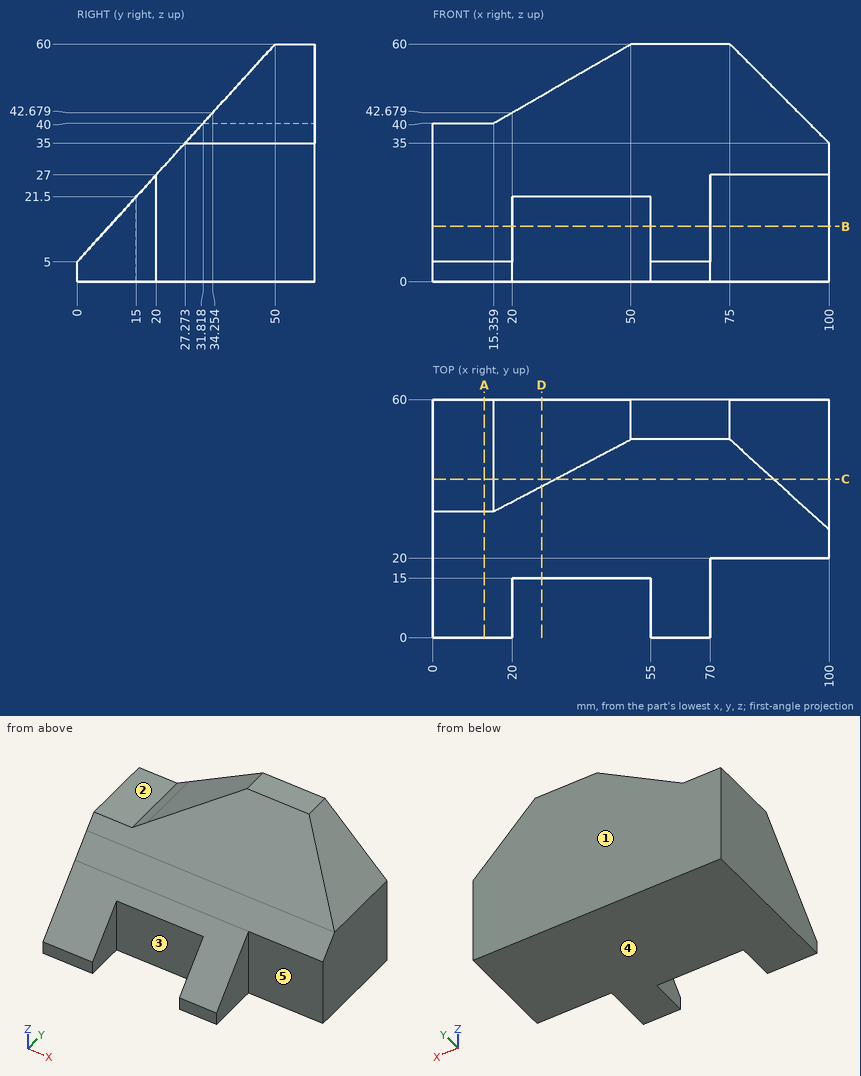
Answer from the drawing. Dimensions are ordinates in mm from the lowest x, y and z of the part. A direction names the side the tool comes from. Round coordinates to 2 decimals unless told otherwise and drop trailing zeros. Write each loop counter-clockwise with the first axis right and the second up, starting at its lowest first coordinate (ties: lowest second). Pieces come first, ordered by that corner, then holes. Notation, with made-up numbers: (-7.5, -16) -> (29.5, -16) arc R29 cw to (29.5, 11) -> close; hole circle Ø1 at (88.5, 51.5). An arc over 180 degrees is marked (long way). Answer in a Markdown table with one row per item. Add a question column.
1) Find section D-D, the plane x = 27.5. Determine the outline of the cut face in (y, z), and give its area (3 significant figures).
2) Given P1, Ø5, axis at x = 10.5, y = 19.5, coming from the -Z side; P2, Ø8, axis at x = 83.5, z = 15.5, coming from the -Y side; P3, Ø2, axis at x = 24.5, y = 18, coming from the +Z side; P4, Ø4.5, axis at x = 9.5, y = 43, coming from the +Z side, each flat-ended and moving along its own axis, determine where each tip first touches the part or whether it passes through.
3) Find section B-B, the plane z = 14. Determine the outline of the cut face in (x, y).
4) Find section C-C, the plane y = 40. Determine the outline of the cut face in (x, z), and give its area (3 significant figures).
5) Consider line 1 (Y direction, x = 25, z = 18.5); line 2 (Y direction, x = 33, z = 49); line 3 (Z direction, x = 52, y = 20). Determine where each line is inside the solid, lowest interval first.
6) Find section A-A, the plane x = 13. Determine the outline of the cut face in (y, z), and give its area (3 significant figures).
7) Which of the six approach directions +Z, -Z, +X, -X, +Y, -Y give full straight-line access (tool end or side, diameter ignored) to the marked faces 1, 2, 3, 4 and 5?
Findings below:
| question | item | result |
|---|---|---|
| 1 | outline | (15, 0) -> (60, 0) -> (60, 47.01) -> (38.19, 47.01) -> (15, 21.5) -> close |
| 1 | area | 1,820 mm² |
| 2 | P1 | z = 0 |
| 2 | P2 | y = 20 |
| 2 | P3 | z = 25.9 |
| 2 | P4 | z = 40 |
| 3 | outline | (0, 8.18) -> (20, 8.18) -> (20, 15) -> (55, 15) -> (55, 8.18) -> (70, 8.18) -> (70, 20) -> (100, 20) -> (100, 60) -> (0, 60) -> close |
| 4 | outline | (0, 0) -> (100, 0) -> (100, 35) -> (86, 49) -> (30.95, 49) -> (15.36, 40) -> (0, 40) -> close |
| 4 | area | 4,590 mm² |
| 5 | line 1 | 15 to 60 |
| 5 | line 2 | 40 to 60 |
| 5 | line 3 | 0 to 27 |
| 6 | outline | (0, 0) -> (60, 0) -> (60, 40) -> (31.82, 40) -> (0, 5) -> close |
| 6 | area | 1,840 mm² |
| 7 | face 1 | +Z, -Z, +X, -X, +Y |
| 7 | face 2 | +Z, -X, +Y, -Y |
| 7 | face 3 | +Z, -Z, -Y |
| 7 | face 4 | -Z, +X, -X, +Y, -Y |
| 7 | face 5 | +Z, -Z, +X, -Y |
